The listing builds one solid part. Answer for the finished solid, in the listing's coordinates (mm). A direction names the side the tool comes from. Coordinates: 2 decimals unless noted, no trailing zeros. Order: outer loops, then holes, each group sorted by start corner. A loop starts at its lowest first (then second) coordinate and runs counter-clockwise, first axis right, second up. Notation, with made-up numbers: (62.25, -7) -> (71.25, -7) arc R23 ccw to (71.25, 32) -> close; hole circle Ø9 at (0, -24). An arc over 180 degrees is marked (long way). Return JSON: item names as keys, results as strings.
from build123d import *

# Parameters (mm, degrees)
SKETCH1_R   = 6.35
SKETCH1_R_2 = 5.995762211


with BuildPart() as part:
    # Sweep1: sweep along a path in Sketch2
    with BuildLine(Plane(origin=(0, 0, 0), x_dir=(0, 0, -1), z_dir=(1, 0, 0))) as sweep1_path:
        Line((0, 0), (0, 38.1))
        ThreePointArc((0, 38.1), (-1.763384176, 49.556890961), (-6.890307113, 59.953262225))
        Line((-6.890307113, 59.953262225), (-50.596831563, 122.372648))
        ThreePointArc((-50.596831563, 122.372648), (-55.723754499, 132.769019264), (-57.487138675, 144.225910225))
        Line((-57.487138675, 144.225910225), (-57.487138675, 195.025910225))
    # Sketch1 → Sweep1 (sweep)
    with BuildSketch(Plane(origin=(0, 0, 0), x_dir=(1, 0, 0), z_dir=(0, 1, 0))):
        Circle(SKETCH1_R)
        Circle(SKETCH1_R_2, mode=Mode.SUBTRACT)
    sweep(path=sweep1_path.line)


solid = part.part
1. For faces 1 (the face through (-0.781, 19.317, -5.945)), 2 (the face through (-1.377, 169.982, 63.686)), 3 (the face through (-0.78, 95.01, 24.18)), determine the directions among +Z, -Z, +X, -X, +Y, -Y from which every point of the face is accessible in a straight line to the end or side of a thin tool.
Answer block:
{"face 1": "-Y", "face 2": "+Y", "face 3": "none"}
2. Consider line 1 (X direction, y = 27, z = 0); line 2 (Z direction, x = 0, y = 177). Determine where each line is inside the solid, lowest interval first. Write a range as from..to.
Answer block:
{"line 1": "x = -6.35..-6, 6..6.35", "line 2": "z = 51.14..51.49, 63.48..63.84"}
3. The part is cut by section B-B on y = 36. Give the vertices of the cut face in (x, z).
Answer block:
{"outline": "circle Ø12.7 at (0, 0); hole circle Ø11.99 at (0, 0)"}
4. Determine the mould class of faces 4 (the face through (-1.377, 88.044, 34.127)), 5 (the face through (-1.3, 169.98, 63.34)) for opening direction X: pulls with the +X half, pulls with the -X half, needs draft (parallel to the pull), parting line crosses it, or undercut.
Answer block:
{"face 4": "parting line crosses it", "face 5": "undercut"}
5. Each of these flat-tipped pins is pushed along its axis until it touches: pin 1 Ø5 at (x, y) = (1.5, 92.5) entering from +Z; pin 2 Ø3 at (x, y) = (-0.5, 59) entering from -Z; pin 3 Ø4 at (x, z) = (1, 43.5) entering from +Y. Where does it stop, or does it pass through?
Answer block:
{"pin 1": "stops at z = 39.05", "pin 2": "stops at z = -1.88", "pin 3": "stops at y = 126.07"}
6. The part is cut by section A-A on x = 0. Give the vertices of the cut face in (y, z), and give its area (3 significant figures).
Answer block:
{"outline": "(0, -6.35) -> (38.1, -6.35) arc R44.45 ccw to (63.6, 1.69) -> (126.01, 45.4) arc R31.75 cw to (144.23, 51.14) -> (195.03, 51.14) -> (195.03, 51.49) -> (144.23, 51.49) arc R32.1 ccw to (125.81, 45.69) -> (63.39, 1.98) arc R44.1 cw to (38.1, -6) -> (0, -6) -> close; (0, 6) -> (38.1, 6) arc R32.1 ccw to (56.51, 11.8) -> (118.93, 55.51) arc R44.1 cw to (144.23, 63.48) -> (195.03, 63.48) -> (195.03, 63.84) -> (144.23, 63.84) arc R44.45 ccw to (118.73, 55.8) -> (56.31, 12.09) arc R31.75 cw to (38.1, 6.35) -> (0, 6.35) -> close", "area": "150 mm2"}
